Verification items for the finished model (mm, model axes). A direction names the side the tool comes from. Coordinates: 2 decimals unless noted, no trailing zeros. Loops run counter-clockwise (first coordinate to the right, second up) from the corner with the lowest first, then second, coordinate; pieces in that order, holes last. Notation, with made-up numbers: (17.25, 56) - (75.25, 56) arc R17 ccw to (75.25, 83) - close; hole circle Ø10 at (-12, 76.25). An arc over 180 degrees is marked (long way). One line per item, written item: value. Start each with the question number.
(1) Thickness scan on probe 1 along Y at (x, z) = (0, 16); probe 2 along Y at (x, z) = (0, 24); probe 3 along Z at (x, y) = (-12, -12). Record the ranges inside material, lowest first. Write a range as [from, to].
(2) Gauge pin test, flat ends, axial feed: P1, Ø5, axis at y = -16, z = 18, coming from the -X side; P2, Ø14, axis at x = -4.5, y = -2.5, coming from the +Z side; P3, Ø6, axis at x = 18.5, y = -15, coming from the -Z side; P4, Ø10, axis at y = -10, z = 25.5, coming from the +X side. Record the tip position at first contact, or that the pin passes through.
(3) Section check D-D (x = 15). Record the boundary of the cut face in (y, z), plus the area to 3 significant figures.
(4) Draft check along X on faces 4 (the face through (19, -19, 31.5)), 5 (the face through (-19.46, 17.84, 24.84)), 6 (the face through (-5.506, 24.796, 7.395)). Enter one of: +X half, -X half, draft (parallel to the pull), parting line (faces both ways), or undercut.
(5) Section check C-C (z = 23.5). Record the boundary of the cut face in (x, y).
(6) Section check A-A (y = 0). Record the boundary of the cut face in (x, z), plus the area to 3 significant figures.
(7) Set-up check for faces 1 (the face through (5.3, 0.4, 0)), 2 (the face through (-21, -15, 15)), 3 (the face through (0, 6, 9)): record each of +Z, -Z, +X, -X, +Y, -Y from which the full face is reachable in a straight line by a thin tool's end or side.
Autodesk Inventor part; units mm, degrees
ref_plane "YZ Plane" through (0, 0, 0) normal (1, 0, 0) x (0, 1, 0)
ref_plane "XZ Plane" through (0, 0, 0) normal (0, 1, 0) x (-1, 0, 0)
ref_plane "XY Plane" through (0, 0, 0) normal (0, 0, 1) x (1, 0, 0)
sketch "Sketch1" plane through (0, 0, 0) normal (0, 0, 1) x (1, 0, 0)
  circle A0 centre (0, 0) radius 25.4
  dimension "d0" = 50.8
extrude "Extrusion1" add sketch "Sketch1" along normal blind 15
sketch "Sketch2" plane through (0, 0, 15) normal (0, 0, 1) x (1, 0, 0)
  circle A0 centre (0, 0) radius 25.4
  circle A1 centre (0, 0) radius 28.4
  dimension "d3" = 56.8
extrude "Extrusion2" add sketch "Sketch2" along normal blind 16.5 contours A0 | A1
sketch "Sketch3" plane through (0, 0, 31.5) normal (0, 0, 1) x (1, 0, 0)
  circle A0 centre (0, 0) radius 28.4
  circle A1 centre (0, 0) radius 26.4
  dimension "d6" = 52.8
extrude "Extrusion3" cut sketch "Sketch3" against normal blind 13.5 contours A1
sketch "Sketch4" plane through (0, 0, 18) normal (0, 0, 1) x (1, 0, 0)
  circle A0 centre (0, 0) radius 26.4
  circle A1 centre (0, 0) radius 23.4
  dimension "d9" = 46.8
extrude "Extrusion4" cut sketch "Sketch4" against normal blind 9 contours A1
sketch "Sketch5" plane through (0, 0, 9) normal (0, 0, 1) x (1, 0, 0)
  circle A0 centre (0, 0) radius 23.4
  circle A1 centre (0, 0) radius 5
  dimension "d12" = 10
extrude "Extrusion5" cut sketch "Sketch5" against normal through all contours A1
properties part number "PZTmount"
Responses:
1. probe 1: y = [-28.4, -23.4], [23.4, 28.4]
1. probe 2: y = [-28.4, -26.4], [26.4, 28.4]
1. probe 3: z = [0, 9]
2. P1: stops at x = -24.99
2. P2: stops at z = 9
2. P3: stops at z = 0
2. P4: stops at x = 27.96
3. outline: (-24.12, 15) - (-20.5, 15) - (-20.5, 0) - (20.5, 0) - (20.5, 15) - (24.12, 15) - (24.12, 31.5) - (21.72, 31.5) - (21.72, 18) - (17.96, 18) - (17.96, 9) - (-17.96, 9) - (-17.96, 18) - (-21.72, 18) - (-21.72, 31.5) - (-24.12, 31.5) - close
3. area: 501 mm²
4. face 4: draft
4. face 5: undercut
4. face 6: parting line
5. outline: circle Ø56.8 at (0, 0); hole circle Ø52.8 at (0, 0)
6. outline: (-28.4, 15) - (-25.4, 15) - (-25.4, 0) - (-5, 0) - (-5, 9) - (-23.4, 9) - (-23.4, 18) - (-26.4, 18) - (-26.4, 31.5) - (-28.4, 31.5) - close; (5, 0) - (25.4, 0) - (25.4, 15) - (28.4, 15) - (28.4, 31.5) - (26.4, 31.5) - (26.4, 18) - (23.4, 18) - (23.4, 9) - (5, 9) - close
6. area: 475 mm²
7. face 1: -Z, +X, -X, +Y, -Y
7. face 2: -Z
7. face 3: +Z
